Could you check a few things on this drawing? It's one solid part, dimensions in mm from its lowest x, y, z. A direction names the side the tool comes from. Give positions to 0.01 mm unless a question says otherwise; leave off trailing zeros. Order: outer loops, then holes, each group sorted by start corner. A loop starts at its lowest first (then second) coordinate and runs counter-clockwise, first axis right, second up. Notation, with made-up numbers: (34.5, -39) -> (71.5, -39) arc R16 cw to (71.5, -14) -> close; hole circle Ø2 at (-0.75, -35.75). An arc over 180 degrees is marked (long way). Write each question's results on one line, items separated by ' | '.
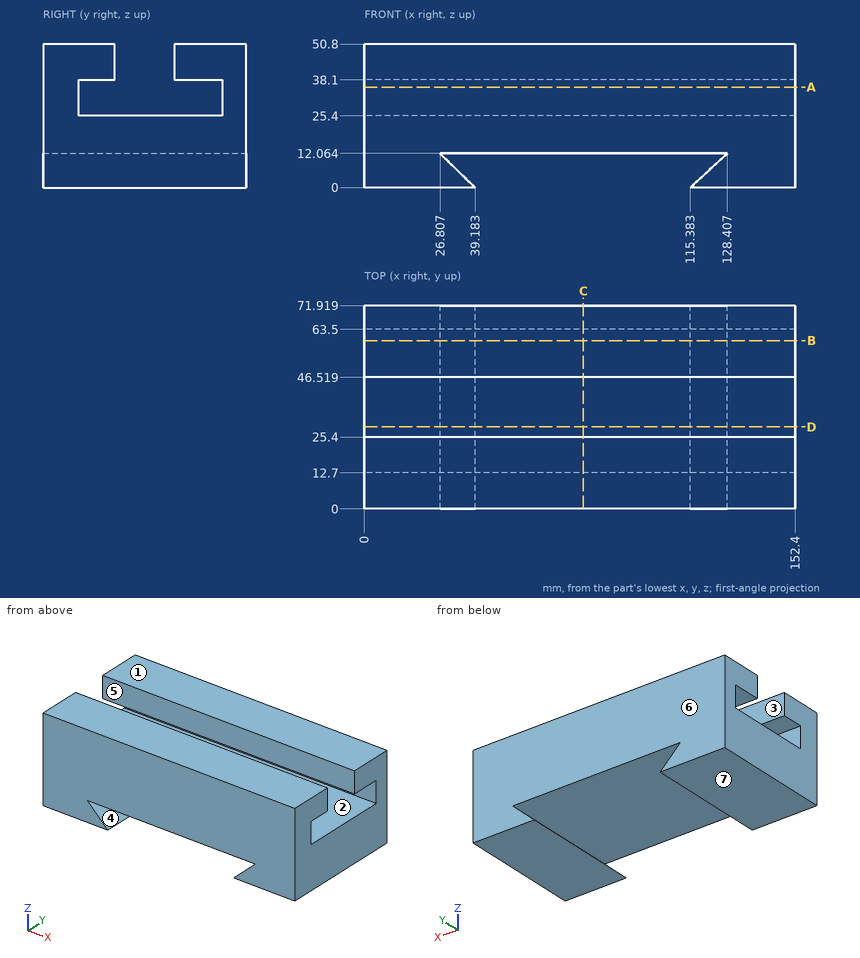
Q1. Suppose I cut it at B-B on y = 59.5. Please give me the cut outline in (x, z) (1 decimal).
Here are the results:
outline: (0, 0) -> (39.2, 0) -> (26.8, 12.1) -> (128.4, 12.1) -> (115.4, 0) -> (152.4, 0) -> (152.4, 25.4) -> (0, 25.4) -> close; (0, 38.1) -> (152.4, 38.1) -> (152.4, 50.8) -> (0, 50.8) -> close
Q2. I need wall thicknesses on line 1 along Y through (x, z) = (34.5, 42.5); line 2 along Z through (x, y) = (38, 47.5) (1 decimal); line 3 along Z through (x, y) = (139.5, 51). Which ranges of each line are inside material? Lowest first, please.
Here are the results:
line 1: y = 0 to 25.4, 46.52 to 71.92 | line 2: z = 0 to 1.2, 12.1 to 25.4, 38.1 to 50.8 | line 3: z = 0 to 25.4, 38.1 to 50.8
Q3. For the marked faces 1, 2, 3 and 4, which set-ups out of +Z, -Z, +X, -X, +Y, -Y let a thin tool reach every point of the face, with its end or its side?
Here are the results:
face 1: +Z, +X, -X, +Y, -Y | face 2: +X, -X | face 3: +Z, +X, -X | face 4: +Y, -Y
Q4. I'm going to push a flat-ended pin straight in: pin 1 Ø10 at (x, y) = (65.5, 21.5) entering from -Z. Where does the tip first touch, or does it pass through?
Here are the results:
pin 1: stops at z = 12.06
Q5. Thinking about a two-plate mould opening in Y: for the marked faces 5, 6 and 7, which applies, +Y half, -Y half, draft (parallel to the pull), parting line (faces both ways), or undercut?
Here are the results:
face 5: undercut | face 6: +Y half | face 7: draft
Q6. Suppose I cut it at A-A on z = 35.5. Please give me the cut outline in (x, y).
Here are the results:
outline: (0, 0) -> (152.4, 0) -> (152.4, 12.7) -> (0, 12.7) -> close; (0, 63.5) -> (152.4, 63.5) -> (152.4, 71.92) -> (0, 71.92) -> close
Q7. Suppose I cut it at D-D on y = 29. Please give me the cut outline in (x, z) (1 decimal).
Here are the results:
outline: (0, 0) -> (39.2, 0) -> (26.8, 12.1) -> (128.4, 12.1) -> (115.4, 0) -> (152.4, 0) -> (152.4, 25.4) -> (0, 25.4) -> close
Q8. Suppose I cut it at C-C on x = 77.5. Please give me the cut outline in (y, z) (1 decimal).
Here are the results:
outline: (0, 12.1) -> (71.9, 12.1) -> (71.9, 50.8) -> (46.5, 50.8) -> (46.5, 38.1) -> (63.5, 38.1) -> (63.5, 25.4) -> (12.7, 25.4) -> (12.7, 38.1) -> (25.4, 38.1) -> (25.4, 50.8) -> (0, 50.8) -> close
